Autodesk Inventor part; units mm, degrees
ref_plane "Work Plane1" through (-15, 0, -53) normal (-1, 0, 0) x (0, 0, 1)
ref_plane "YZ Plane" through (0, 0, 0) normal (1, 0, 0) x (0, 1, 0)
ref_plane "XZ Plane" through (0, 0, 0) normal (0, 1, 0) x (-1, 0, 0)
sketch "Sketch1" plane through (0, 0, 0) normal (0, 1, 0) x (-1, 0, 0)
  line L0 (0, 0) -> (30, 0)
  line L1 (30, 0) -> (30, -53)
  line L2 (30, -53) -> (0, -53)
  line L3 (0, -53) -> (0, 0)
  dimension "d0" = 30
  dimension "d1" = 53
extrude "Extrusion1" add sketch "Sketch1" along normal blind 5
sketch "Sketch2" plane through (0, 5, 0) normal (0, 1, 0) x (1, 0, 0)
  line L0 (-30, 53) -> (-30, 0)
  line L1 (0, 53) -> (-30, 53)
  line L2 (-30, 53) -> (-30, 39)
  line L3 (-30, 39) -> (0, 39)
  line L4 (0, 39) -> (0, 53)
  line L5 (0, 0) -> (-30, 0)
  line L6 (-30, 0) -> (-30, 14)
  line L7 (-30, 14) -> (0, 14)
  line L8 (0, 14) -> (0, 0)
  line L9 (0, 39) -> (-30, 39)
  line L10 (-30, 39) -> (-30, 14)
  line L11 (-30, 14) -> (0, 14)
  line L12 (0, 14) -> (0, 39)
  dimension "d4" = 14
  dimension "d5" = 14
extrude "Extrusion2" add sketch "Sketch2" along normal blind 8 contours L3 L12 L7 L0
sketch "Sketch3" plane through (0, 13, 0) normal (0, 1, 0) x (1, 0, 0)
  circle A0 centre (-15, 26.5) radius 7.5
  point P0 (0, 0)
  dimension "d8" = 15
extrude "Extrusion3" add sketch "Sketch3" along normal blind 3
ref_plane "Work Plane1" through (-15, 0, -53) normal (-1, 0, 0) x (0, 0, 1)
sketch "Sketch4" plane through (-15, 0, -53) normal (-1, 0, 0) x (0, 0, 1)
  line L0 (19, 16) -> (26.5, 16)
  line L1 (14, 5) -> (14, 13)
  line L2 (39, 5) -> (39, 13)
  line L3 (53, 0) -> (0, 0)
  line L4 (53, 0) -> (53, 5)
  line L5 (39, 5) -> (53, 5)
  line L6 (39, 5) -> (39, 13)
  line L7 (14, 13) -> (39, 13)
  line L8 (14, 5) -> (14, 13)
  line L9 (0, 5) -> (14, 5)
  line L10 (0, 0) -> (0, 5)
  line L11 (26.5, 16) -> (14, 16)
  line L12 (26.5, 16) -> (26.5, 21)
  arc A0 (21.1584, 21) -> (14, 16) centre (20.9681, 13.6482) ccw
  line L13 (21.1584, 21) -> (26.5, 21)
revolve "Revolution1" add sketch "Sketch4" angle 360 about axis through (-15, 16, -26.5) along (0, 1, 0) contours L11 A0 L13 L12 L0
sketch "Sketch5" plane through (0, 5, 0) normal (0, 1, 0) x (1, 0, 0)
  line L0 (-6.6727, 10.5436) -> (-23.7046, 10.5436)
  line L1 (-23.7046, 3.3179) -> (-6.6727, 3.3179)
  arc A0 (-6.6727, 3.3179) -> (-6.6727, 10.5436) centre (-6.6727, 6.9307) ccw
  arc A1 (-23.7046, 10.5436) -> (-23.7046, 3.3179) centre (-23.7046, 6.9307) ccw
  line L2 (0, 14) -> (0, 39)
  line L3 (0, 26.5) -> (-37.5908, 26.5)
  line L4 (-6.6727, 42.4564) -> (-23.7046, 42.4564)
  line L5 (-23.7046, 49.6821) -> (-6.6727, 49.6821)
  arc A2 (-6.6727, 42.4564) -> (-6.6727, 49.6821) centre (-6.6727, 46.0693) ccw
  arc A3 (-23.7046, 49.6821) -> (-23.7046, 42.4564) centre (-23.7046, 46.0693) ccw
  point P0 (0, 0)
extrude "Extrusion4" cut sketch "Sketch5" against normal blind 32
fillet "Fillet1" radius 0.5 10 edges at (0, 5, -7) (-30, 5, -7) (-15, 5, 0) (0, 5, -46) (-15, 5, -53) (-30, 5, -46) (-30, 2.5, -53) (-30, 2.5, 0) (0, 2.5, 0) (0, 2.5, -53)
fillet "Fillet2" radius 1.5 2 edges at (-15, 13, -14) (-15, 13, -39)
properties part number "button"
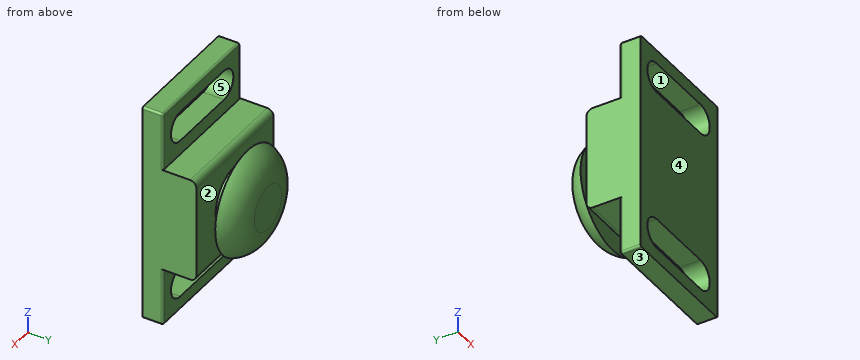
Model file for the job. Use its own axes, mm. Face numbers are marked on the shaded views. A direction names the side the tool comes from. Give positions to 0.01 mm unless a question says otherwise; leave off trailing zeros. Loops run counter-clockwise (first coordinate to the right, second up) from the corner with the lowest first, then second, coordinate; pieces in that order, holes last.
Item 1: Slice it at A-A (y = 2.75). Write the cut outline in (x, z), plus the area to 3 significant figures.
Check values:
outline: (-30, -52.5) arc R0.5 ccw to (-29.5, -53) - (-0.5, -53) arc R0.5 ccw to (0, -52.5) - (0, -0.5) arc R0.5 ccw to (-0.5, 0) - (-29.5, 0) arc R0.5 ccw to (-30, -0.5) - close; hole (-23.7, -49.68) - (-6.67, -49.68) arc R3.61 ccw to (-6.67, -42.46) - (-23.7, -42.46) arc R3.61 ccw to start; hole (-23.7, -10.54) - (-6.67, -10.54) arc R3.61 ccw to (-6.67, -3.32) - (-23.7, -3.32) arc R3.61 ccw to start
area: 1,260 mm2
Item 2: Slice it at C-C (x = -15). Give the number of separate pieces and of enclosed holes in the cut face, plus the area to 3 significant figures.
Check values:
separate pieces: 3
enclosed holes: 0
area: 543 mm2
Item 3: Slice it at B-B (z = -43.5). Write the cut outline in (x, y), plus the area to 3 significant figures.
Check values:
outline: (-30, 0) - (-26.24, 0) - (-26.24, 5) - (-29.5, 5) arc R0.5 ccw to (-30, 4.5) - close; (-4.13, 0) - (0, 0) - (0, 4.5) arc R0.5 ccw to (-0.5, 5) - (-4.13, 5) - close
area: 39.3 mm2
Item 4: Slice it at D-D (z = -4). Write the cut outline in (x, y).
Check values:
outline: (-30, 0) - (-25.82, 0) - (-25.82, 5) - (-29.5, 5) arc R0.5 ccw to (-30, 4.5) - close; (-4.56, 0) - (0, 0) - (0, 4.5) arc R0.5 ccw to (-0.5, 5) - (-4.56, 5) - close
Item 5: Mould opens along Z. For the marked faces 1, 2 and 3 say: +Z half, -Z half, draft (parallel to the pull), parting line (faces both ways), or undercut.
Check values:
face 1: undercut
face 2: draft
face 3: -Z half
Item 6: Drop flat-ended pins along their axis: P1, Ø4, axis at x = -19, z = -10.5, coming from the +Y side; P2, Ø8.5, axis at x = -16, z = -25.5, coming from the +Y side; P3, Ø4, axis at x = -21, y = 10, coming from the -Z side; P4, Ø3, axis at x = -8, z = -45.5, coming from the +Y side. Give the stop position or say it passes through.
Check values:
P1: stops at y = 5
P2: stops at y = 21
P3: stops at z = -39
P4: passes through
Item 7: Which spindle directions (+Z, -Z, +X, -X, +Y, -Y) get a long thin tool onto all of the face, cutting with end or side? Do the marked faces 4 and 5. Say none if no direction does.
Check values:
face 4: +Z, -Z, +X, -X, -Y
face 5: +Y, -Y
Item 8: Drill centre lines: line 1 along Z through (x, y) = (-14, 1.5); line 2 along Z through (x, y) = (-26.5, 3); line 3 along Y through (x, z) = (-3.25, -47.5). Where is each one in solid material? Low to high.
Check values:
line 1: z = -53 to -49.68, -42.46 to -10.54, -3.32 to 0
line 2: z = -53 to -48.36, -43.78 to -9.22, -4.64 to 0
line 3: y = 0 to 5
